The listing builds one solid part. Answer for the finished solid, in the listing's coordinates (mm). A direction names the side the tool comes from. Give positions to 0.01 mm unless a question says otherwise; leave off trailing zeros. Order: outer loops, then holes, each group sorted by start corner. A loop starts at its lowest first (then second) coordinate and runs counter-clockwise, first axis right, second up. Notation, with made-up numbers: (-4.75, 79.25) - (49.25, 79.25) arc R37 ccw to (49.25, 116.25) - close; hole circle Ø7 at (57, 26.25). An arc over 180 degrees is marked (long way). Answer in a Markdown table with one row per item. Add a question column.
```python
from build123d import *

# Parameters (mm, degrees)
F0_W     = 140
F0_H     = 140
F1_DEPTH = 5
F2_SIZE  = 2
F3_R     = 21
F3_R_2   = 19
F4_DEPTH = 80
F5_R     = 5


with BuildPart() as f1:
    # F0 (on Top) → F1 (new body)
    with BuildSketch(Plane.XY):
        Rectangle(F0_W, F0_H)
    extrude(amount=F1_DEPTH)

    # F2
    f2_edges = [f1.edges().sort_by_distance(p)[0] for p in [
        (0, -70, 5),
        (0, 70, 5),
        (-70, 0, 5),
        (70, 0, 5),
    ]]
    chamfer(f2_edges, length=F2_SIZE)

    # F3 (on face) → F4 (join)
    with BuildSketch(Plane.XY.offset(5)):
        with Locations((-35, 30)):
            Circle(F3_R)
        with Locations((35, 30)):
            Circle(F3_R)
        with Locations((-35, -35)):
            Circle(F3_R_2)
        with Locations((35, -35)):
            Circle(F3_R_2)
    extrude(amount=F4_DEPTH)

    # F5
    f5_edges = [f1.edges().sort_by_distance(p)[0] for p in [
        (-56, 30, 85),
        (14, 30, 85),
        (-54, -35, 85),
        (16, -35, 85),
    ]]
    fillet(f5_edges, radius=F5_R)


solid = f1.part
```
(1) Find section D-D, the plane y = -35. Write down the section's boundary in (x, z).
(2) Find section A-A, the plane y = 30. Write down the section's boundary in (x, z).
(3) Straight lines are drawn through the part: line 1 (Y direction, x = -36, z = 9); line 2 (X direction, y = -36, z = 73.5); line 3 (Z direction, x = 47, y = 51.5). For each, find the intervals that lie inside material, in ascending order.
(4) For faces 1 (the face through (35, -35, 85)), 2 (the face through (-1, 1, 5)), determine the directions among +Z, -Z, +X, -X, +Y, -Y from which every point of the face is accessible in a straight line to the end or side of a thin tool.
(5) Find section C-C, the plane x = 1.5. Write down the section's boundary in (y, z), plus the area to 3 significant figures.
(6) Each of these flat-tipped pins is pushed along its axis until it touches: P1, Ø10, axis at y = 20.5, z = 11, coming from the +X side; P2, Ø4, axis at y = -37, z = 30, coming from the -X side; P3, Ø4, axis at y = 38, z = 61.5, coming from the +X side. Where does it stop, or does it pass through?
(7) Find section B-B, the plane z = 60. Write down the section's boundary in (x, y).
(8) The mould has two halves that part along X. Classify faces 3 (the face through (-35, 30, 85)), 4 (the face through (46.3, 47.7, 42)): +X half, -X half, draft (parallel to the pull), parting line (faces both ways), or undercut.
Answer key:
| question | item | result |
|---|---|---|
| 1 | outline | (-70, 0) - (70, 0) - (70, 3) - (68, 5) - (54, 5) - (54, 80) arc R5 ccw to (49, 85) - (21, 85) arc R5 ccw to (16, 80) - (16, 5) - (-16, 5) - (-16, 80) arc R5 ccw to (-21, 85) - (-49, 85) arc R5 ccw to (-54, 80) - (-54, 5) - (-68, 5) - (-70, 3) - close |
| 2 | outline | (-70, 0) - (70, 0) - (70, 3) - (68, 5) - (56, 5) - (56, 80) arc R5 ccw to (51, 85) - (19, 85) arc R5 ccw to (14, 80) - (14, 5) - (-14, 5) - (-14, 80) arc R5 ccw to (-19, 85) - (-51, 85) arc R5 ccw to (-56, 80) - (-56, 5) - (-68, 5) - (-70, 3) - close |
| 3 | line 1 | -53.97 to -16.03, 9.02 to 50.98 |
| 3 | line 2 | -53.97 to -16.03, 16.03 to 53.97 |
| 3 | line 3 | 0 to 5 |
| 4 | face 1 | +Z, +X, -X, +Y, -Y |
| 4 | face 2 | +Z |
| 5 | outline | (-70, 0) - (70, 0) - (70, 3) - (68, 5) - (-68, 5) - (-70, 3) - close |
| 5 | area | 696 mm² |
| 6 | P1 | x = 55.51 |
| 6 | P2 | x = -54 |
| 6 | P3 | x = 55.12 |
| 7 | outline | circle Ø42 at (-35, 30); circle Ø38 at (-35, -35); circle Ø42 at (35, 30); circle Ø38 at (35, -35) |
| 8 | face 3 | draft |
| 8 | face 4 | undercut |
